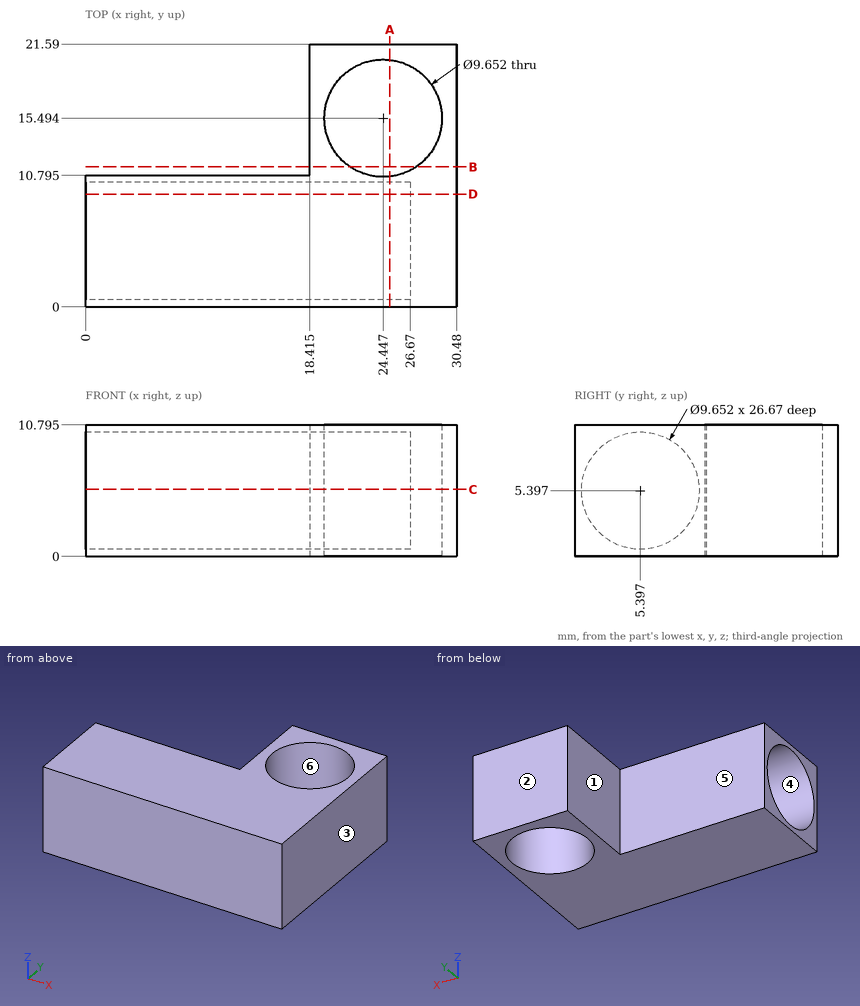
For this review, use the dimensioned drawing (mm, ordinates from the lowest corner) and the shaded views. A direction names the side the tool comes from. Give positions to 0.01 mm unless a question says otherwise; leave off trailing zeros. Order: outer loops, then holes, each group sorted by start corner. A loop starts at its lowest first (then second) coordinate and runs counter-clockwise, first axis right, second up.
1) For the marked faces 1 and 2, list the 3-axis set-ups (+Z, -Z, +X, -X, +Y, -Y) from which the entire face can be reached by the end or side of a thin tool; tool diameter is ignored.
2) Insertion check: pin 1 (3 mm diameter, centred on y = 5.5, z = 7, fed in from -X); pin 2 (5.5 mm diameter, centred on y = 18.5, z = 7, fed in from -X) (1 decimal); pin 3 (1 mm diameter, centred on x = 5, z = 7, fed in from +Y) (1 decimal). Each pin has a flat end and moves straight along its axis. Give the tip position at first contact, or say it passes through.
3) Take a section at A-A (x = 25). Give the boundary of the cut face in (y, z) (1 decimal).
4) The part is to be moulded in two halves that separate along Y. For the marked faces 3, 4, 5 and 6, say which applies: released by +Y, released by -Y, zero draft, split by the parting line, or undercut.
5) Take a section at D-D (y = 9.25). Give the boundary of the cut face in (x, z) (1 decimal), then the cut area to 3 significant figures.
6) Take a section at C-C (z = 5.5). Give the boundary of the cut face in (x, y) (1 decimal), then the cut area to 3 significant figures.
7) Wall thickness on line 1 (Y direction, x = 26, z = 3) (1 decimal); line 2 (X direction, y = 6.75, z = 5.75); line 3 (Y direction, x = 19.5, z = 5.5): over which ranges is each line inside the solid? List them lowest first.
8) Take a section at B-B (y = 11.5). Give the boundary of the cut face in (x, z) (1 decimal).
Derived:
1. face 1: +Z, -Z, -X, +Y
1. face 2: +Z, -Z, +X, -X, +Y
2. pin 1: stops at x = 26.67
2. pin 2: stops at x = 18.4
2. pin 3: stops at y = 10.8
3. outline: (0, 0) - (10.7, 0) - (10.7, 10.8) - (0, 10.8) - close; (20.3, 0) - (21.6, 0) - (21.6, 10.8) - (20.3, 10.8) - close; hole circle Ø9.7 at (5.4, 5.4)
4. face 3: zero draft
4. face 4: undercut
4. face 5: released by +Y
4. face 6: undercut
5. outline: (0, 0) - (30.5, 0) - (30.5, 10.8) - (0, 10.8) - (0, 8.3) - (26.7, 8.3) - (26.7, 2.5) - (0, 2.5) - close
5. area: 174 mm2
6. outline: (0, 0) - (30.5, 0) - (30.5, 21.6) - (18.4, 21.6) - (18.4, 10.8) - (0, 10.8) - (0, 10.2) - (26.7, 10.2) - (26.7, 0.6) - (0, 0.6) - close; hole circle Ø9.7 at (24.4, 15.5)
6. area: 129 mm2
7. line 1: y = 0 to 1.2, 9.6 to 10.9, 20.1 to 21.6
7. line 2: x = 26.67 to 30.48
7. line 3: y = 0 to 0.57, 10.22 to 21.59
8. outline: (18.4, 0) - (21.7, 0) - (21.7, 10.8) - (18.4, 10.8) - close; (27.2, 0) - (30.5, 0) - (30.5, 10.8) - (27.2, 10.8) - close
